Input: part model. Units: mm. Frame: model coordinates. A direction names the side the tool comes from. Give positions to 0.01 mm unless a question says otherwise; leave off trailing zeros. Loops run counter-clockwise (first coordinate to the right, second up) from the corner with the lowest first, then second, coordinate; pieces in that order, holes last. Notation, with made-up numbers: (-37, 70) - (-18, 70) arc R13 ccw to (-18, 81) - close; hole circle Ø1 at (-14, 4). An arc over 180 degrees is marked (long way). One line per item, written item: value.
Autodesk Inventor part; units mm, degrees
ref_plane "YZ Plane" through (0, 0, 0) normal (1, 0, 0) x (0, 1, 0)
ref_plane "XZ Plane" through (0, 0, 0) normal (0, 1, 0) x (-1, 0, 0)
ref_plane "XY Plane" through (0, 0, 0) normal (0, 0, 1) x (1, 0, 0)
sketch "Sketch1" plane through (0, 0, 0) normal (0, 1, 0) x (-1, 0, 0)
  line L0 (277.6855, 25.4) -> (-277.6855, 25.4)
  line L1 (-277.6855, 25.4) -> (-277.6855, -25.4)
  line L2 (-277.6855, -25.4) -> (277.6855, -25.4)
  line L3 (277.6855, -25.4) -> (277.6855, 25.4)
  line L4 (277.6855, 25.4) -> (-277.6855, -25.4) construction
  line L5 (-277.6855, 25.4) -> (277.6855, -25.4) construction
  point P0 (0, 0)
  dimension "d0" = 555.371
  dimension "d1" = 50.8
extrude "Extrusion1" add sketch "Sketch1" along normal blind 3.048
sketch "Sketch2" plane through (-277.6855, 0, 25.4) normal (0, 0, 1) x (1, 0, 0)
  line L0 (0, 0) -> (555.371, 0)
  line L1 (555.371, 0) -> (428.371, 0)
  line L2 (555.371, 0) -> (555.371, -73.3235)
  line L3 (555.371, -73.3235) -> (428.371, 0)
  line L4 (0, 0) -> (127, 0)
  line L5 (127, 0) -> (0, -73.3235)
  line L6 (0, -73.3235) -> (0, 0)
  point P0 (277.6855, 0)
  dimension "d6" = 127
  dimension "d8" = 127
  dimension "d9" = 30
  dimension "d15" = 30
extrude "Extrusion2" add sketch "Sketch2" against normal blind 25.4 contours L0 L2 L3
extrude "Extrusion3" add sketch "Sketch2" against normal blind 25.4 contours L0 L5 L6
sketch "Sketch3" plane through (0, 0, 0) normal (0, -1, 0) x (1, 0, 0)
  line L0 (-277.6855, 25.4) -> (277.6855, 25.4) construction
  line L1 (-277.6855, 25.4) -> (0, 25.4) construction
  line L2 (0, 0) -> (0, 25.4) construction
  line L3 (184.15, 25.4) -> (-184.15, 25.4)
  line L4 (-184.15, 25.4) -> (-184.15, 0)
  line L5 (-184.15, 0) -> (184.15, 0)
  line L6 (184.15, 0) -> (184.15, 25.4)
  line L7 (184.15, 25.4) -> (-184.15, 0) construction
  line L8 (-184.15, 25.4) -> (184.15, 0) construction
  point P0 (0, 12.7)
  dimension "d16" = 368.3
extrude "Extrusion4" add sketch "Sketch3" along normal blind 19.05
equation "\"d6\" = d8"
equation "\"d15\" = d9"
properties part number "Wire Housing Lid vglue"
Item 1: Draft query along X for faces 4 (the face through (-277.686, -36, 12)), 5 (the face through (-3, -19.05, 13)), 6 (the face through (-1, -9, 0)). Return one class per face: pulls with the +X half, pulls with the -X half, needs draft (parallel to the pull), parting line crosses it, or undercut.
Verdict:
face 4: pulls with the -X half
face 5: undercut
face 6: needs draft
Item 2: Section A-A, the plane y = -36.5. Output: boundary loops of the cut face in (x, z).
Verdict:
outline: (-277.69, 0) - (-213.91, 0) - (-213.91, 25.4) - (-277.69, 25.4) - close; (213.91, 0) - (277.69, 0) - (277.69, 25.4) - (213.91, 25.4) - close
Item 3: Access query for faces 1 (the face through (4, 0, -13)), 2 (the face through (-230.03, -45.81, 12.88)), 3 (the face through (277.686, -36, 12)). Directions: +Z, -Z, +X, -X, +Y, -Y. A direction counts if a zero-diameter tool reaches every point of the face in a straight line with its end or side. Return the directions, or none.
Verdict:
face 1: -Z, +X, -X, -Y
face 2: +Z, -Z, -Y
face 3: +Z, -Z, +X, +Y, -Y
Item 4: Section D-D, the plane y = -61.5. Output: boundary loops of the cut face in (x, z), and give its area (3 significant figures).
Verdict:
outline: (-277.69, 0) - (-257.21, 0) - (-257.21, 25.4) - (-277.69, 25.4) - close; (257.21, 0) - (277.69, 0) - (277.69, 25.4) - (257.21, 25.4) - close
area: 1,040 mm^2
Item 5: Section C-C, the plane z = 6. Output: boundary loops of the cut face in (x, y), and give its area (3 significant figures).
Verdict:
outline: (-277.69, -73.32) - (-183.68, -19.05) - (183.68, -19.05) - (277.69, -73.32) - (277.69, 3.05) - (-277.69, 3.05) - close
area: 17,400 mm^2
Item 6: Pin query (flat end, axial travel): P1, Ø20.5, axis at x = 113, z = -15.5, coming from the -Y side; P2, Ø1, axis at x = -80.5, y = -10.5, coming from the -Z side. Return the tip coordinate at first contact, or that it passes through.
Verdict:
P1: stops at y = 0
P2: stops at z = 0
Item 7: Section B-B, the plane x = 50.5. Output: boundary loops of the cut face in (y, z), and give its area (3 significant figures).
Verdict:
outline: (-19.05, 0) - (0, 0) - (0, -25.4) - (3.05, -25.4) - (3.05, 25.4) - (-19.05, 25.4) - close
area: 639 mm^2
Item 8: Material intervals for L1, parallel to Y at x = -118.5, z = 18; L2, parallel to Y at x = 176, z = -18; L3, parallel to X at y = -69, z = 17, sorted ascending.
Verdict:
L1: y = -19.05 to 3.05
L2: y = 0 to 3.05
L3: x = -277.69 to -270.2, 270.2 to 277.69
